Read the model definition and answer for the solid it produces. Units are mm, in the model's axes. A direction names the side the tool comes from. Coordinates: 2 decimals unless noted, no trailing zeros. Order: outer loops, then holes, each group sorted by start corner. A loop starts at its lowest first (then second) coordinate and runs counter-clockwise, first axis right, second up.
from build123d import *
from build123d import SkipClean  # not in build123d's __all__

# Parameters (mm, degrees)
F0_W     = 20
F0_H     = 11.5
F1_DEPTH = 16
F2_W     = 3
F2_H     = 11.5
F3_DEPTH = 25
F4_W     = 17
F4_H     = 7.5
F4_W_2   = 14
F4_H_2   = 5
F5_DEPTH = 10
F6_DEPTH = 25
F7_SIZE2 = 1.0503113073
F7_SIZE  = 1.5
F8_R     = 1


# Not quite as in the source:
# - ends of sketch curves that miss each other by under 0.0002 mm in the source are joined


with BuildPart() as f1:
    # F0 (on Front) → F1 (new body)
    with BuildSketch(Plane.XZ):
        Rectangle(F0_W, F0_H)
        Polygon((13.9961953573, -5.7499998733), (10, -5.7499998733), (-10, -5.75), (-14.0038046427, -5.7499998733), (-14.0038046427, -7.7499998733), (13.9961953573, -7.7499998733), align=None)
    extrude(amount=-F1_DEPTH)

    # F2 (on face) → F3 (cut)
    with BuildSketch(Plane.YZ.offset(10)):
        with Locations((1.5, 0)):
            Rectangle(F2_W, F2_H)
        with Locations((14.50000076, 0)):
            Rectangle(F2_W, F2_H)
    with SkipClean():  # cleaning this boolean's faces spoils the solid; the shape is the same uncleaned
        extrude(amount=-F3_DEPTH, mode=Mode.SUBTRACT)

    # F4 (on face) → F5 (cut)
    with BuildSketch(Plane(origin=(0, 0, -7.7499998733), x_dir=(1, 0, 0), z_dir=(0, 0, -1))):
        with Locations((0, -7.8641947285)):
            Rectangle(F4_W, F4_H)
        with Locations((0, -7.8641947285)):
            Rectangle(F4_W_2, F4_H_2, mode=Mode.SUBTRACT)
    with SkipClean():  # cleaning this boolean's faces spoils the solid; the shape is the same uncleaned
        extrude(amount=-F5_DEPTH, mode=Mode.SUBTRACT)

    # F4 (on face) → F6 (cut)
    with BuildSketch(Plane(origin=(0, 0, -7.7499998733), x_dir=(1, 0, 0), z_dir=(0, 0, -1))):
        with Locations((0, -7.8641947285)):
            Rectangle(F4_W_2, F4_H_2)
    with SkipClean():  # cleaning this boolean's faces spoils the solid; the shape is the same uncleaned
        extrude(amount=-F6_DEPTH, mode=Mode.SUBTRACT)

    # F7
    f7_edges = [f1.edges().sort_by_distance(p)[0] for p in [
        (-0.003805, 16, -7.75),
        (13.996195, 8, -7.75),
        (-0.003805, 0, -7.75),
        (-14.003805, 8, -7.75),
    ]]
    f7_side = f1.faces().sort_by_distance((-13.681314, 8, -7.75))[0]
    chamfer(f7_edges, length=F7_SIZE, length2=F7_SIZE2, reference=f7_side)

    # F8
    f8_edges = [f1.edges().sort_by_distance(p)[0] for p in [
        (10, 3, 0),
        (10, 13.000001, 0),
        (-10, 3, 0),
        (-10, 13.000001, 0),
    ]]
    fillet(f8_edges, radius=F8_R)


solid = f1.part
Q1. The part is cut by section D-D, the plane y = 2. Determine the outline of the cut face in (x, z), then the cut area to 3 significant figures.
Q2. The part is cut by section A-A, the plane x = 2. Determine the outline of the cut face in (y, z), then the cut area to 3 significant figures.
Q3. Which of the six approach directions +Z, -Z, +X, -X, +Y, -Y give full straight-line access (tool end or side, diameter ignored) to faces 4 (the flat face through (0, 4.114, -3)), 5 (the flat face through (-7, 8, 4)), 6 (the flat face through (10, 8, 0)), 7 (the cylindrical face through (9.699, 12.715, 0.08))?
Q4. Each of these flat-tipped pins is pushed along its axis until it touches: P1, Ø1.2, axis at x = 5, y = 1, coming from the +Z side; P2, Ø6, axis at x = -2.5, z = 1.5, coming from the -Y side; P3, Ø1.7, axis at y = 8.5, z = 4.5, coming from the +X side. Where does it stop, or does it pass through?
Q5. The part is cut by section C-C, the plane z = -3.25. Determine the outline of the cut face in (x, y), then the cut area to 3 significant figures.
Q6. Straight lines are drawn through the part: L1, parallel to X at y = 4.75, z = -4; L2, parallel to Y at x = 4.75, z = -3.25; L3, parallel to X at y = 10, z = 5. For each, find the intervals that lie inside material, in ascending order.
Q7. Determine the mould class of faces 1 (the flat face through (0, 5, 2.25)), 2 (the flat face through (0, 3, 0)), 3 (the flat face through (0, 12, -7.75)) for opening direction Y: +Y half, -Y half, draft (parallel to the pull), parting line (faces both ways), or undercut.
Q8. The part is cut by section B-B, the plane y = 6. Determine the outline of the cut face in (x, z).
Computed values:
1. outline: (-14, -6.7) - (-12.5, -7.75) - (12.5, -7.75) - (14, -6.7) - (14, -5.75) - (-14, -5.75) - close
1. area: 54.4 mm2
2. outline: (0, -6.7) - (1.5, -7.75) - (4.11, -7.75) - (4.11, 2.25) - (5.36, 2.25) - (5.36, 5.75) - (3, 5.75) - (3, -5.75) - (0, -5.75) - close; (10.36, 2.25) - (11.61, 2.25) - (11.61, -7.75) - (14.5, -7.75) - (16, -6.7) - (16, -5.75) - (13, -5.75) - (13, 5.75) - (10.36, 5.75) - close
2. area: 52.9 mm2
3. face 4: -Z
3. face 5: +Z, -Z
3. face 6: +Z, +X, +Y, -Y
3. face 7: +Z, +X, +Y
4. P1: stops at z = -5.75
4. P2: stops at y = 3
4. P3: stops at x = 10
5. outline: (-10, 4) arc R1 ccw to (-9, 3) - (9, 3) arc R1 ccw to (10, 4) - (10, 12) arc R1 ccw to (9, 13) - (-9, 13) arc R1 ccw to (-10, 12) - close; hole (-8.5, 4.11) - (8.5, 4.11) - (8.5, 11.61) - (-8.5, 11.61) - close
5. area: 71.6 mm2
6. L1: x = -10 to -8.5, 8.5 to 10
6. L2: y = 3 to 4.11, 11.61 to 13
6. L3: x = -10 to -7, 7 to 10
7. face 1: undercut
7. face 2: -Y half
7. face 3: draft
8. outline: (-14, -6.7) - (-12.5, -7.75) - (-8.5, -7.75) - (-8.5, 2.25) - (-7, 2.25) - (-7, 5.75) - (-10, 5.75) - (-10, -5.75) - (-14, -5.75) - close; (7, 2.25) - (8.5, 2.25) - (8.5, -7.75) - (12.5, -7.75) - (14, -6.7) - (14, -5.75) - (10, -5.75) - (10, 5.75) - (7, 5.75) - close
